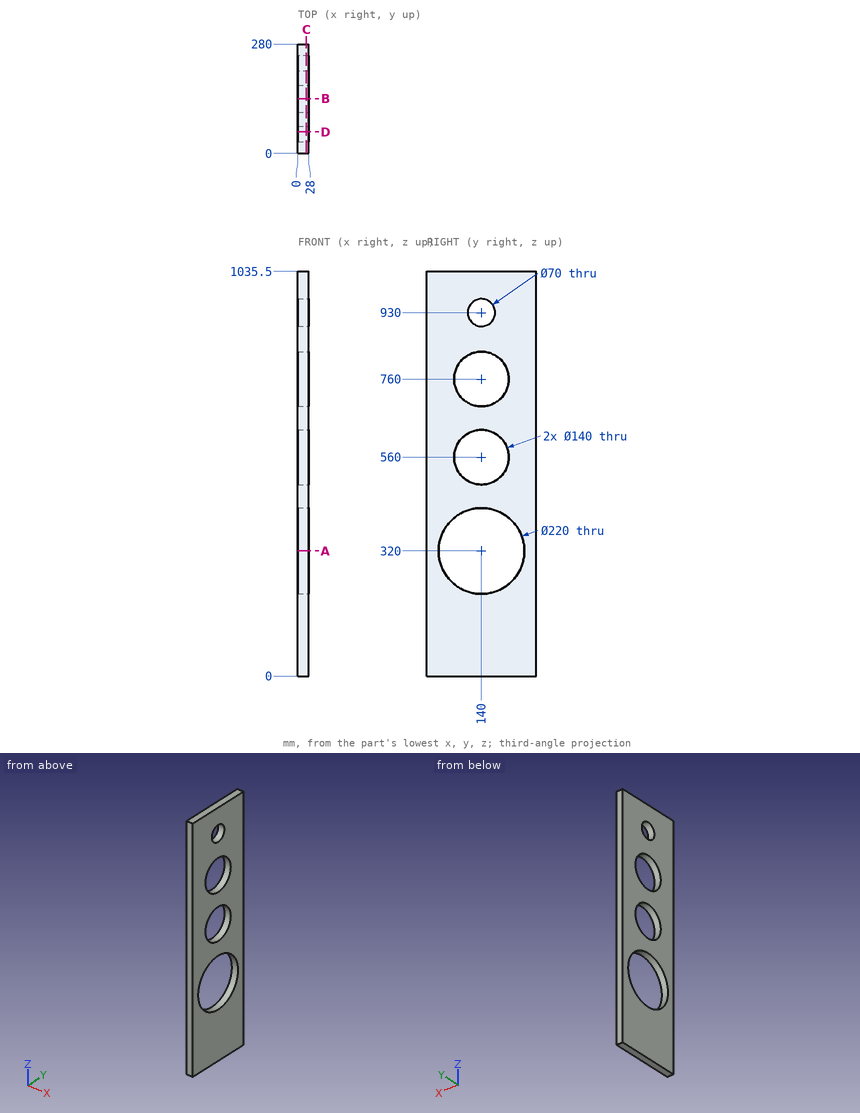
Can you work these out from the drawing? Everything is in mm from the part's minimum corner. Coordinates: 2 decimals unless noted, no trailing zeros. Loops run counter-clockwise (first coordinate to the right, second up) from the corner with the lowest first, then second, coordinate; pieces in that order, holes last.
1) Please list where these lines run through material, in increasing order: line 1 along Z through (x, y) = (11.5, 137); line 2 along Z through (x, y) = (10, 140); line 3 along Y through (x, z) = (7.5, 760).
Reported:
line 1: z = 0 to 210.04, 429.96 to 490.06, 629.94 to 690.06, 829.94 to 895.13, 964.87 to 1035.5
line 2: z = 0 to 210, 430 to 490, 630 to 690, 830 to 895, 965 to 1035.5
line 3: y = 0 to 70, 210 to 280
2) Imagine slicing it at C-C (x = 22). List the corners of the cut face in (y, z) for me, and give its area (3 significant figures).
Reported:
outline: (0, 0) - (280, 0) - (280, 1035.5) - (0, 1035.5) - close; hole circle Ø220 at (140, 320); hole circle Ø140 at (140, 560); hole circle Ø140 at (140, 760); hole circle Ø70 at (140, 930)
area: 217,000 mm2
3) Imagine slicing it at A-A (z = 320). List the corners of the cut face in (x, y) for me.
Reported:
outline: (0, 0) - (28, 0) - (28, 30) - (0, 30) - close; (0, 250) - (28, 250) - (28, 280) - (0, 280) - close
4) Imagine slicing it at D-D (y = 55). List the corners of the cut face in (x, z) for me, and give its area (3 significant figures).
Reported:
outline: (0, 0) - (28, 0) - (28, 250.18) - (0, 250.18) - close; (0, 389.82) - (28, 389.82) - (28, 1035.5) - (0, 1035.5) - close
area: 25,100 mm2
5) Imagine slicing it at B-B (y = 140). List the corners of the cut face in (x, z) for me, and give its area (3 significant figures).
Reported:
outline: (0, 0) - (28, 0) - (28, 210) - (0, 210) - close; (0, 430) - (28, 430) - (28, 490) - (0, 490) - close; (0, 630) - (28, 630) - (28, 690) - (0, 690) - close; (0, 830) - (28, 830) - (28, 895) - (0, 895) - close; (0, 965) - (28, 965) - (28, 1035.5) - (0, 1035.5) - close
area: 13,000 mm2
